Autodesk Inventor part; units mm, degrees
ref_plane "YZ Plane" through (0, 0, 0) normal (1, 0, 0) x (0, 1, 0)
ref_plane "XZ Plane" through (0, 0, 0) normal (0, 1, 0) x (-1, 0, 0)
ref_plane "XY Plane" through (0, 0, 0) normal (0, 0, 1) x (1, 0, 0)
sketch "Náčrt1" plane through (0, 0, 0) normal (0, 0, 1) x (1, 0, 0)
  line L0 (0, 33.6) -> (0, -33.6)
  line L1 (-11.7, 0) -> (31.7, 0)
  line L2 (-2.5, -24) -> (2.5, -24)
  line L3 (2.5, -24) -> (2.5, 4.6603)
  line L4 (2.5, 4.6603) -> (11.9338, 21)
  line L5 (11.9338, 21) -> (25.5, 21)
  line L6 (25.5, 21) -> (25.5, 24)
  line L7 (25.5, 24) -> (-5.5, 24)
  line L8 (-5.5, 24) -> (-5.5, 21)
  line L9 (-5.5, 21) -> (11.9338, 21)
  line L10 (-2.5, -24) -> (-2.5, 6)
  line L11 (-2.5, 6) -> (6.1603, 21)
  point P0 (0, 0)
  dimension "d0" = 5
  dimension "d2" = 5
  dimension "d3" = 30
  dimension "d4" = 15
  dimension "d5" = 31
  dimension "d6" = 3
  dimension "d7" = 60
  dimension "d8" = 3
extrude "Vysunutí1" add sketch "Náčrt1" along normal blind 15 contours L7 L6 L5 L9 L0 | L0 L9 L8 L7 | L11 L9 L4 L3 L1 L0 | L0 L1 L10 L11 | L1 L3 L2 L0 | L0 L2 L10 L1
sketch "Náčrt2" plane through (-2.5, -24, 0) normal (-1, 0, 0) x (0, 0, 1)
  line L0 (0, 30) -> (0, 0)
  line L1 (0, 0) -> (15, 0)
  line L2 (15, 30) -> (15, 0)
  line L3 (0, 30) -> (15, 30)
  line L4 (0, -9.6) -> (0, 57.6)
  line L5 (-3, 24) -> (18, 24)
  point P0 (0, 24)
  point P1 (7.5, 15)
  dimension "d11" = 15
  dimension "d12" = 7.5
hole "Díra1" at (-2.5, -9, 7.5) direction (1, 0, 0) diameter 6.6 end through all
sketch "Náčrt3" plane through (-5.5, 24, 0) normal (0, 1, 0) x (1, 0, 0)
  line L0 (31, 0) -> (0, 0)
  line L1 (0, 0) -> (0, -15)
  line L2 (31, -15) -> (0, -15)
  line L3 (31, 0) -> (31, -15)
  line L4 (5.5, 3) -> (5.5, -18)
  line L5 (37.2, 0) -> (-6.2, 0)
  point P0 (5.5, 0)
  point P1 (24, -7.5)
  point P2 (31, -7.5)
  dimension "d20" = 7.5
  dimension "d21" = 7
hole "Díra2" at (18.5, 24, 7.5) direction (0, -1, 0) diameter 3.3 end through all
fillet "Zaoblení1" radius 2 4 edges at (11.9338, 21, 7.5) (6.1603, 21, 7.5) (2.5, 4.6603, 7.5) (-2.5, 6, 7.5)
sketch "Náčrt4" plane through (0, 0, 0) normal (0, 0, -1) x (-1, 0, 0)
  arc A0 (2.5, 5.4641) -> (2.2321, 6.4641) centre (0.5, 5.4641) ccw
  line L0 (-4.4282, 18) -> (2.2321, 6.4641)
  arc A1 (-2.6962, 21) -> (-4.4282, 18) centre (-2.6962, 19) ccw
  line L1 (5.5, 21) -> (-2.6962, 21)
  line L2 (5.5, 24) -> (5.5, 21)
  line L3 (-25.5, 24) -> (5.5, 24)
  line L4 (-25.5, 21) -> (-25.5, 24)
  line L5 (-13.0885, 21) -> (-25.5, 21)
  arc A2 (-11.3564, 20) -> (-13.0885, 21) centre (-13.0885, 19) ccw
  line L6 (-2.7679, 5.1244) -> (-11.3564, 20)
  arc A3 (-2.5, 4.1244) -> (-2.7679, 5.1244) centre (-4.5, 4.1244) ccw
  line L7 (-2.5, -24) -> (-2.5, 4.1244)
  line L8 (2.5, -24) -> (-2.5, -24)
  line L9 (2.5, 5.4641) -> (2.5, -24)
  line L10 (2.5, -14) -> (-2.5, -14)
  line L11 (-2.5, -14) -> (-2.5, -4)
  line L12 (-2.5, -4) -> (2.5, -4)
  line L13 (2.5, -4) -> (2.5, -14)
  point P0 (0, 0)
  dimension "d30" = 10
  dimension "d31" = 10
extrude "Vysunutí2" add sketch "Náčrt4" along normal blind 15 contours L9 L10 L7 L12
properties part number "IR_senzor_hold_v2_3D tisk"
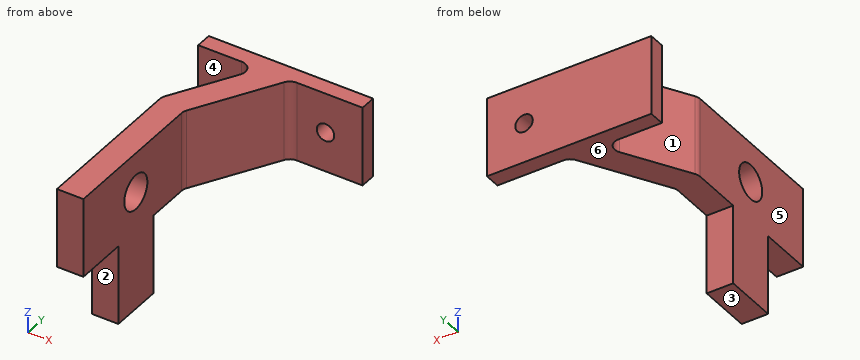
Could you check a few things on this model? Use its own coordinates, in mm. Face numbers are marked on the shaded views. A direction names the side the tool comes from. Coordinates: 2 decimals unless noted, no trailing zeros. Loops run counter-clockwise (first coordinate to the right, second up) from the corner with the lowest first, then second, coordinate; pieces in that order, holes last.
1. For P1, Ø7.5, axis at y = -9, z = 7.5, coming from the +X side; P2, Ø4, axis at x = 1, z = -5.5, coming from the -Y side; P3, Ø2.5, axis at x = 0.5, z = -5, coming from the +Y side; P4, Ø1, axis at x = 4.5, z = -6.5, coming from the -Y side, each with a flat end and sliding along its axis, tell me the tip position at first contact or that it passes through.
2. Imagine slicing it at B-B (y = -9). Please give me the cut outline in (x, z).
3. Imagine slicing it at D-D (z = 12.25). Please give me the cut outline in (x, y), and give its area (3 significant figures).
4. I need wall thicknesses on L1, parallel to X at y = 22.35, z = 7.5; L2, parallel to Z at x = 0, y = -9; L3, parallel to Y at x = 0, z = 7.5. Which ranges of each line are inside material? Lowest first, please.
5. Imagine slicing it at A-A (z = 7.5). Please give me the cut outline in (x, y), and give its area (3 significant figures).
6. For the marked faces 4, 5 and 6, which set-ups out of +Z, -Z, +X, -X, +Y, -Y let a thin tool reach every point of the face, with its end or its side?
7. Imagine slicing it at C-C (x = 18.5). Please give me the cut outline in (y, z), and give its area (3 significant figures).
8. We'd pull the mould along Y, two halves only. Please class the marked faces 1, 2 and 3: released by +Y, released by -Y, zero draft, split by the parting line, or undercut.
Computed values:
1. P1: stops at x = 2.5
1. P2: stops at y = -14
1. P3: stops at y = -4
1. P4: passes through
2. outline: (-2.5, -15) - (2.5, -15) - (2.5, 4.2) - (-2.5, 4.2) - close; (-2.5, 10.8) - (2.5, 10.8) - (2.5, 15) - (-2.5, 15) - close
3. outline: (-5.5, 21) - (2.7, 21) arc R2 cw to (4.43, 18) - (-2.23, 6.46) arc R2 ccw to (-2.5, 5.46) - (-2.5, -24) - (2.5, -24) - (2.5, 4.12) arc R2 cw to (2.77, 5.12) - (11.36, 20) arc R2 cw to (13.09, 21) - (25.5, 21) - (25.5, 24) - (-5.5, 24) - close
3. area: 333 mm2
4. L1: x = -5.5 to 16.85, 20.15 to 25.5
4. L2: z = -15 to 4.2, 10.8 to 15
4. L3: y = -24 to -12.3, -5.7 to 10.33, 21 to 24
5. outline: (-5.5, 21) - (2.7, 21) arc R2 cw to (4.43, 18) - (-2.23, 6.46) arc R2 ccw to (-2.5, 5.46) - (-2.5, -5.7) - (2.5, -5.7) - (2.5, 4.12) arc R2 cw to (2.77, 5.12) - (11.36, 20) arc R2 cw to (13.09, 21) - (16.85, 21) - (16.85, 24) - (-5.5, 24) - close; (-2.5, -24) - (2.5, -24) - (2.5, -12.3) - (-2.5, -12.3) - close; (20.15, 21) - (25.5, 21) - (25.5, 24) - (20.15, 24) - close
5. area: 290 mm2
6. face 4: +Z, -Z, -X
6. face 5: +Z, -Z, -X, -Y
6. face 6: -Z, +X, -X, +Y
7. outline: (21, 0) - (24, 0) - (24, 5.85) - (21, 5.85) - close; (21, 9.15) - (24, 9.15) - (24, 15) - (21, 15) - close
7. area: 35.1 mm2
8. face 1: undercut
8. face 2: released by -Y
8. face 3: zero draft
